Check sheet for the modelled part. Datum: model origin and axes. Units: mm. A direction names the side the tool comes from. Give positions to 0.01 mm unless a question says otherwise; leave off trailing zeros. Order: outer loops, then holes, each group sorted by start corner. A loop starts at its lowest first (then second) coordinate and runs counter-clockwise, first axis right, second up.
from build123d import *

# Parameters (mm, degrees)
F0_R     = 120.65
F0_W     = 9.525
F0_H     = 25.4
F0_R_2   = 10.31875
F1_DEPTH = 7.9375


with BuildPart() as f1:
    # F0 (on Top) → F1 (new body)
    with BuildSketch(Plane.XY):
        Circle(F0_R)
        with Locations((-69.05625, -44.45)):
            Rectangle(F0_W, F0_H, mode=Mode.SUBTRACT)
        with Locations((70.64375, -44.45)):
            Rectangle(F0_W, F0_H, mode=Mode.SUBTRACT)
        with Locations((-69.05625, 44.45)):
            Rectangle(F0_W, F0_H, mode=Mode.SUBTRACT)
        Circle(F0_R_2, mode=Mode.SUBTRACT)
        with Locations((70.64375, 44.45)):
            Rectangle(F0_W, F0_H, mode=Mode.SUBTRACT)
    extrude(amount=F1_DEPTH)


solid = f1.part
1) Depth check by flat-ended pin: pin 1 Ø10 at (x, y) = (-35, -31) entering from -Z; pin 2 Ø2.5 at (y, z) = (-42.5, 3) entering from +X; pin 3 Ø4 at (x, z) = (-69.5, 2.5) entering from -Y; pin 4 Ø2.5 at (y, z) = (41, 4.5) entering from -X. Enter the tip coordinate at first touch or a pass-through.
Recorded:
pin 1: stops at z = 0
pin 2: stops at x = 113.38
pin 3: stops at y = -100
pin 4: stops at x = -113.91
2) Section check D-D, the plane y = -40. Record the cut outline in (x, z).
Recorded:
outline: (-113.83, 0) - (-73.82, 0) - (-73.82, 7.94) - (-113.83, 7.94) - close; (-64.29, 0) - (65.88, 0) - (65.88, 7.94) - (-64.29, 7.94) - close; (75.41, 0) - (113.83, 0) - (113.83, 7.94) - (75.41, 7.94) - close
3) Draft check along Y on faces 3 (the face through (75.406, 44, 4)), 4 (the face through (-2, -25, 0)), 5 (the face through (-120.533, 5.305, 3.913)). Enter one of: +Y half, -Y half, draft (parallel to the pull), parting line (faces both ways), or undercut.
Recorded:
face 3: undercut
face 4: draft
face 5: parting line
4) Section check B-B, the plane z = 2.25. Record the cut outline in (x, y), then the cut area to 3 significant figures.
Recorded:
outline: circle Ø241.3 at (0, 0); hole (-73.82, -57.15) - (-64.29, -57.15) - (-64.29, -31.75) - (-73.82, -31.75) - close; hole (-73.82, 31.75) - (-64.29, 31.75) - (-64.29, 57.15) - (-73.82, 57.15) - close; hole circle Ø20.64 at (0, 0); hole (65.88, -57.15) - (75.41, -57.15) - (75.41, -31.75) - (65.88, -31.75) - close; hole (65.88, 31.75) - (75.41, 31.75) - (75.41, 57.15) - (65.88, 57.15) - close
area: 44,400 mm2
5) Section check A-A, the plane x = 0. Record the cut outline in (y, z), then the cut area to 3 significant figures.
Recorded:
outline: (-120.65, 0) - (-10.32, 0) - (-10.32, 7.94) - (-120.65, 7.94) - close; (10.32, 0) - (120.65, 0) - (120.65, 7.94) - (10.32, 7.94) - close
area: 1,750 mm2
6) Set-up check for faces 1 (the face through (-2, -25, 7.938)), 2 (the face through (-69, -31.75, 4)): record each of +Z, -Z, +X, -X, +Y, -Y from which the full face is reachable in a straight line by a thin tool's end or side.
Recorded:
face 1: +Z, +X, -X, +Y, -Y
face 2: +Z, -Z
7) Material ranges on L1, parallel to Y at x = 0, z = 5.5; L2, parallel to X at y = -37.5, z = 5.75; L3, parallel to X at y = 56.5, z = 7.25, recorded low to high.
Recorded:
L1: y = -120.65 to -10.32, 10.32 to 120.65
L2: x = -114.67 to -73.82, -64.29 to 65.88, 75.41 to 114.67
L3: x = -106.6 to -73.82, -64.29 to 65.88, 75.41 to 106.6
